The model under review builds one solid part; all positions refer to its coordinate system, in mm. Face numbers are marked on the shaded views. A direction names the side the tool comes from. Coordinates: 2 decimals unless noted, no trailing zeros. Loops run counter-clockwise (first coordinate to the right, second up) from the corner with the lowest first, then second, coordinate; pieces in that order, holes last. Notation, with made-up numbers: M -38,-11.5 L -33,-11.5 A32 cw -33,21.5 Z; hole C 14,-3 d8. An arc over 180 degrees is marked long. One line per item, written item: value.
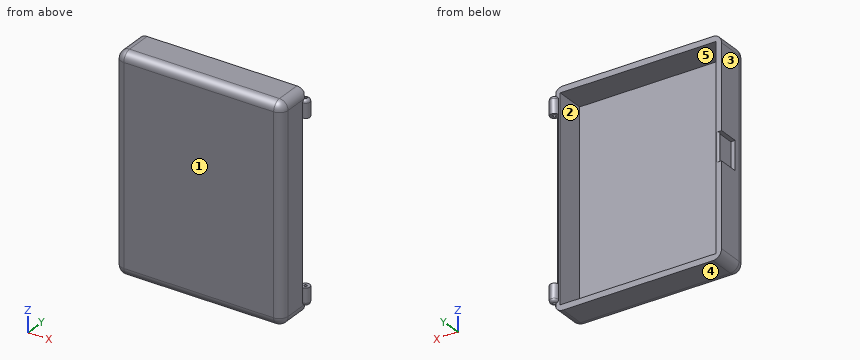
```python
from build123d import *

# Parameters (mm, degrees)
BOTTOM_W                 = 58
BOTTOM_H                 = 74
BOTTOM_W_2               = 54
BOTTOM_H_2               = 70
DUVAR_DEPTH              = 12
BOTTOM_2_W               = 54
BOTTOM_2_H               = 70
TABAN_DEPTH              = 2
FILLET2_R                = 3
MENTESE_OUT_R            = 1.5
MENTESE_DEPTH            = 68
MENTESE_DELIK_DEPTH      = 93.355292214
MENTESE_DELIK_DEPTH_BACK = 93.355292214
MENTESE_IN_R             = 0.5
MENTESE_FILLET_R         = 1
MENTESE_OUT_CUT_R        = 1.5
MENTESE_BOSLUK_DEPTH     = 56
CENTIK_W                 = 1.5
CENTIK_H                 = 10
CENTIK_BOSLUK_DEPTH      = 7
DIL_R                    = 0.5
BOSS_EXTRUDE5_DEPTH      = 10


with BuildPart() as part:
    # bottom → duvar (new body)
    with BuildSketch(Plane(origin=(0, 0, 0), x_dir=(1, 0, 0), z_dir=(0, 1, 0))):
        with Locations((27, 35)):
            Rectangle(BOTTOM_W, BOTTOM_H)
        with Locations((27, 35)):
            Rectangle(BOTTOM_W_2, BOTTOM_H_2, mode=Mode.SUBTRACT)
    extrude(amount=DUVAR_DEPTH)

    # bottom<2> → taban (add)
    with BuildSketch(Plane(origin=(0, 0, 0), x_dir=(1, 0, 0), z_dir=(0, 1, 0))):
        with Locations((27, 35)):
            Rectangle(BOTTOM_2_W, BOTTOM_2_H)
    extrude(amount=TABAN_DEPTH)

    # Fillet2
    fillet2_edges = [part.edges().sort_by_distance(p)[0] for p in [
        (27, 0, -72),
        (56, 0, -35),
        (27, 0, 2),
        (-2, 0, -35),
        (-2, 6, -72),
        (56, 6, -72),
        (56, 6, 2),
        (-2, 6, 2),
    ]]
    fillet(fillet2_edges, radius=FILLET2_R)

    # mentese out → mentese (add)
    with BuildSketch(Plane(origin=(0, 0, -69), x_dir=(-1, 0, 0), z_dir=(0, 0, -1))):
        with Locations((-56, 12)):
            Circle(MENTESE_OUT_R)
    extrude(amount=-MENTESE_DEPTH)

    # mentese in → mentese delik (cut, two sides: drawn at the far end of the back side and taken through both)
    with BuildSketch(Plane.XY.offset(-1).offset(-MENTESE_DELIK_DEPTH_BACK)):
        with Locations(Location((56, 12, 0), (0, 0, 270))):
            Circle(MENTESE_IN_R)
    extrude(amount=MENTESE_DELIK_DEPTH + MENTESE_DELIK_DEPTH_BACK, mode=Mode.SUBTRACT)

    # mentese fillet
    mentese_fillet_edges = [part.edges().sort_by_distance(p)[0] for p in [
        (57.060660172, 13.060660172, -69),
        (57.060660172, 13.060660172, -1),
    ]]
    fillet(mentese_fillet_edges, radius=MENTESE_FILLET_R - 0.0001)  # a hair under: the kernel refuses the full size

    # mentese out cut → mentese bosluk (cut)
    with BuildSketch(Plane(origin=(0, 0, -63), x_dir=(-1, 0, 0), z_dir=(0, 0, -1))):
        with Locations((-56, 12)):
            Circle(MENTESE_OUT_CUT_R)
    extrude(amount=-MENTESE_BOSLUK_DEPTH, mode=Mode.SUBTRACT)

    # centik → centik bosluk (cut)
    with BuildSketch(Plane(origin=(0, 12, 0), x_dir=(1, 0, 0), z_dir=(0, 1, 0))):
        with Locations((-1.25, 35)):
            Rectangle(CENTIK_W, CENTIK_H)
    extrude(amount=-CENTIK_BOSLUK_DEPTH, mode=Mode.SUBTRACT)

    # dil → Boss-Extrude5 (add)
    with BuildSketch(Plane.XY.offset(-40)):
        with Locations((-0.5, 11.5)):
            Circle(DIL_R)
    extrude(amount=BOSS_EXTRUDE5_DEPTH)


solid = part.part
```
(1) Tool access review of the marked faces 4 and 5: name each direction out of +Z, -Z, +X, -X, +Y, -Y from which nothing blocks a thin tool from reaching the whole face with its end or side.
Checks:
face 4: -Z, +X, -X, +Y, -Y
face 5: +Y
(2) Add section D-D on z = -46. State the section outline as (x, y) points, then the cut area to 3 significant figures.
Checks:
outline: M -2,3 A3 ccw 1,0 L 53,0 A3 ccw 56,3 L 56,10.5 A1.5 cw 54.5,12 L 54,12 L 54,2 L 0,2 L 0,12 L -2,12 Z
area: 150 mm^2
(3) Add section C-C on x = 32. State the section outline as (y, z) points.
Checks:
outline: M 0,-69 A3 ccw 3,-72 L 12,-72 L 12,-70 L 2,-70 L 2,0 L 12,0 L 12,2 L 3,2 A3 ccw 0,-1 Z
(4) To check wall thickness, follow L1, parallel to X at y = 9.75, z = -19; L2, parallel to Z at x = 2.5, y = 10.5; L3, parallel to X at y = 7.25, z = -37. State the ranges of each line that lie inside material, in increasing order. Write a range as [from, to].
Checks:
L1: [-2, 0], [54, 56]
L2: [-72, -70], [0, 2]
L3: [-0.5, 0], [54, 56]
(5) Insertion check: pin 1 Ø1.6 at (x, y) = (-1.5, 7.5) entering from -Z; pin 2 Ø3 at (y, z) = (9, -42.5) entering from +X; pin 3 Ø6 at (x, z) = (35, -55.5) entering from +Y. Each pin has a flat end and moves straight along its axis. Give the tip position at first contact, or say it passes through.
Checks:
pin 1: z = -71.47
pin 2: x = 56
pin 3: y = 2
(6) Draft analysis for pull direction X (two halves, no side actions). For the marked faces 1, 2 and 3, state which applies: pulls with the +X half, pulls with the -X half, needs draft (parallel to the pull), parting line crosses it, or undercut.
Checks:
face 1: needs draft
face 2: undercut
face 3: pulls with the -X half
(7) Add section A-A on y = 8.5. State the section outline as (x, z) points, then the cut area to 3 significant figures.
Checks:
outline: M -2,-69 A3 ccw 1,-72 L 53,-72 A3 ccw 56,-69 L 56,-1 A3 ccw 53,2 L 1,2 A3 ccw -2,-1 L -2,-30 L -0.5,-30 L -0.5,-40 L -2,-40 Z; hole M 0,-70 L 54,-70 L 54,0 L 0,0 Z
area: 489 mm^2
(8) Add section B-B on z = -37.5. State the section outline as (x, y) points.
Checks:
outline: M -2,3 A3 ccw 1,0 L 53,0 A3 ccw 56,3 L 56,10.5 A1.5 cw 54.5,12 L 54,12 L 54,2 L 0,2 L 0,12 L -0.5,12 A0.5 ccw -0.5,11 L -0.5,5 L -2,5 Z
